Check sheet for the modelled part. Datum: model origin and axes. Units: mm. A direction names the side the tool comes from. Give positions to 0.01 mm unless a question says otherwise; leave off trailing zeros. Loops run counter-clockwise (first coordinate to the right, second up) from the corner with the lowest first, then second, coordinate; pieces in that order, holes last. Notation, with made-up numbers: (51, 18) -> (71, 18) arc R9 cw to (71, 31) -> close; hole circle Ø2 at (23, 40). An arc over 180 degrees is marked (long way). Write each question's results on one line, items separated by ' | '. Start each with the question number.
1. Material ranges on L1, parallel to X at y = 8, z = 2; L2, parallel to Z at x = 13.5, y = -2; L3, parallel to Z at x = 11, y = 3, recorded low to high. Write a range as from..to.
2. Tool access check on faces 1 (the face through (16, -10, 21)), 2 (the face through (11, 0, 40.49)), 3 (the face through (16, 10, 21)), 4 (the face through (16.3, 0, 41)). Record the directions out of +Z, -Z, +X, -X, +Y, -Y that give a thin tool (end or side, any length) a straight path to the whole face; none if there is none.
3. Gauge pin test, flat ends, axial feed: pin 1 Ø1 at (x, y) = (42.5, 11) entering from +Z; pin 2 Ø3 at (y, z) = (3, 29.5) entering from -X; pin 3 Ø1 at (x, y) = (16.5, 7) entering from -Z; pin 4 Ø2 at (y, z) = (3.5, 41) entering from +X. Record the tip position at first contact, or that the pin passes through.
4. Cross-section at B-B on y = 26. Record the boundary of the cut face in (x, z), and give its area (3 significant figures).
5. Cross-section at C-C on z = 55. Record the boundary of the cut face in (x, y).
6. Mould release check, pull along X, two halves, no side actions. Record for faces 5 (the face through (6.156, 0.14, 22.258)), 6 (the face through (24.3, 0.1, 18.8)), 7 (the face through (9, 0, 42.49)): +X half, -X half, draft (parallel to the pull), parting line (faces both ways), or undercut.
7. Cross-section at A-A on x = 14. Record the boundary of the cut face in (y, z).
from build123d import *

# Parameters (mm, degrees)
CYLINDER001_R             = 35
CYLINDER001_DEPTH         = 2
PAD002_DEPTH              = 10
FUSION002_PLACEMENT_ANGLE = 270


with BuildPart() as cilindro_grande:
    # Cylinder001 → Cylinder001 (new body)
    with BuildSketch(Plane(origin=(-16.3, 0, 0), x_dir=(0, 0, -1), z_dir=(1, 0, 0))):
        Circle(CYLINDER001_R)
    extrude(amount=CYLINDER001_DEPTH)


with BuildPart() as obj1:
    # Sketch005 → Pad002 (new body, symmetric)
    with BuildSketch(Plane.XY):
        with BuildLine():
            add(Edge.make_bspline(
                [(-11.28, 8.59), (-12.232885, 7.961762), (-12.561857, 4.634312), (-12.202327, -1.322686), (-10.996973, -7.076074), (-10.262423, -9.386153), (-10, -9.49)],
                knots=[0, 0, 0, 0, 0.25, 0.5, 0.75, 1, 1, 1, 1], degree=3))
            Line((-10, -9.49), (0, -9.49))
            Line((0, -9.49), (0, -11.49))
            Line((0, -11.49), (-14.42, -11.49))
            Line((-14.42, -11.49), (-14.25, 10.48))
            Line((-14.25, 10.48), (30.7825887629, 13.9608816937))
            Line((30.7825887629, 13.9608816937), (30.9357048732, 11.98))
            Line((30.9357048732, 11.98), (-9.04, 8.89))
            Line((-9.04, 8.89), (-11.28, 8.59))
        make_face()
    extrude(amount=PAD002_DEPTH, both=True)

    # Fusion002: union cilindro_grande
    add(cilindro_grande.part)


with BuildPart() as obj1_1:
    # Fusion002 placement: moved
    add(obj1.part.moved(Location((16.3, 0, 31))).rotate(Axis((16.3, 0, 31), (1, 0, 0)), FUSION002_PLACEMENT_ANGLE))


solid = obj1_1.part
Geometry says:
1) L1: 0..2 | L2: 19.63..21.63, 40.49..42.49 | L3: 19.83..21.82, 40.49..42.49
2) face 1: +Z, -Z, +X, -Y | face 2: +X, +Y, -Y | face 3: +Z, -Z, +X, +Y | face 4: +Z, +X, +Y, -Y
3) pin 1: through | pin 2: x = 0 | pin 3: z = 19.36 | pin 4: x = 16.3
4) outline: (0, 7.57) -> (2, 7.57) -> (2, 54.43) -> (0, 54.43) -> close | area: 93.7 mm^2
5) outline: (0, -25.48) -> (2, -25.48) -> (2, 25.48) -> (0, 25.48) -> close
6) face 5: +X half | face 6: undercut | face 7: draft
7) outline: (-10, 19.6) -> (10, 19.6) -> (10, 21.59) -> (-10, 21.59) -> close; (-10, 40.49) -> (10, 40.49) -> (10, 42.49) -> (-10, 42.49) -> close
